from build123d import *

# Parameters (mm, degrees)
SKETCH1_R           = 150.5
BOSS_EXTRUDE1_DEPTH = 6.35
SKETCH3_R           = 2.6
CUT_EXTRUDE2_DEPTH  = 10
CUT_EXTRUDE3_DEPTH  = 10


with BuildPart() as part:
    # Sketch1 → Boss-Extrude1 (new body)
    # profile 1 of 2: a face of its own
    with BuildSketch(Plane(origin=(-388.281715987, 0, -288.185661777), x_dir=(1, 0, 0), z_dir=(0, 1, 0))):
        Polygon((1927.853460271, -13527.084883536), (1965.381699324, -13462.084066777), (1747.570833697, -13084.824581071), (1672.514355591, -13084.824581071), (1454.703489965, -13462.084066777), (1492.231729019, -13527.084883536), align=None)
        with Locations((1710.042594644, -13357.997843795)):
            Circle(SKETCH1_R, mode=Mode.SUBTRACT)
        with BuildLine():
            ThreePointArc((1909.99400131, -13496.418380494), (1909.919076, -13496.98749472), (1910.268520339, -13497.442899434))
            Line((1910.268520339, -13497.442899434), (1927.415821483, -13507.342898365))
            ThreePointArc((1927.415821483, -13507.342898365), (1927.984935702, -13507.417823673), (1928.440340423, -13507.068379346))
            Line((1928.440340423, -13507.068379346), (1948.340338275, -13472.600571997))
            ThreePointArc((1948.340338275, -13472.600571997), (1948.415263583, -13472.031457775), (1948.065819252, -13471.576053055))
            Line((1948.065819252, -13471.576053055), (1930.918518105, -13461.676054122))
            ThreePointArc((1930.918518105, -13461.676054122), (1930.349403886, -13461.601128813), (1929.893999164, -13461.95057314))
            Line((1929.893999164, -13461.95057314), (1909.99400131, -13496.418380494))
        make_face(mode=Mode.SUBTRACT)
        with BuildLine():
            ThreePointArc((1472.019370034, -13471.57605305), (1471.669925699, -13472.031457773), (1471.744851013, -13472.600571998))
            Line((1471.744851013, -13472.600571998), (1491.644848864, -13507.068379347))
            ThreePointArc((1491.644848864, -13507.068379347), (1492.100253585, -13507.41782368), (1492.669367808, -13507.342898369))
            Line((1492.669367808, -13507.342898369), (1509.816668952, -13497.442899438))
            ThreePointArc((1509.816668952, -13497.442899438), (1510.166113284, -13496.987494718), (1510.091187977, -13496.418380495))
            Line((1510.091187977, -13496.418380495), (1490.191190123, -13461.950573141))
            ThreePointArc((1490.191190123, -13461.950573141), (1489.735785404, -13461.60112881), (1489.166671181, -13461.676054117))
            Line((1489.166671181, -13461.676054117), (1472.019370034, -13471.57605305))
        make_face(mode=Mode.SUBTRACT)
        with BuildLine():
            ThreePointArc((1689.392596873, -13114.874577827), (1689.612266763, -13115.404907856), (1690.142596792, -13115.62457775))
            Line((1690.142596792, -13115.62457775), (1729.942592497, -13115.62457775))
            ThreePointArc((1729.942592497, -13115.62457775), (1730.472922528, -13115.404907859), (1730.692592416, -13114.874577827))
            Line((1730.692592416, -13114.874577827), (1730.692592416, -13095.074579966))
            ThreePointArc((1730.692592416, -13095.074579966), (1730.472922526, -13094.544249938), (1729.942592497, -13094.324580043))
            Line((1729.942592497, -13094.324580043), (1690.142596792, -13094.324580043))
            ThreePointArc((1690.142596792, -13094.324580043), (1689.612266761, -13094.544249935), (1689.392596873, -13095.074579966))
            Line((1689.392596873, -13095.074579966), (1689.392596873, -13114.874577827))
        make_face(mode=Mode.SUBTRACT)
    # profile 2 of 2: a face of its own
    with BuildSketch(Plane(origin=(-388.281715987, 0, -288.185661777), x_dir=(1, 0, 0), z_dir=(0, 1, 0))):
        with Locations((1710.042594644, -13357.997843795)):
            Circle(SKETCH1_R)
    extrude(amount=BOSS_EXTRUDE1_DEPTH)

    # Sketch3 → Cut-Extrude2 (cut)
    with BuildSketch(Plane(origin=(0, 6.35, 0), x_dir=(1, 0, 0), z_dir=(0, 1, 0))):
        with Locations(Location((1183.987460829, -12990.268662147, 0), (0, 0, 270))):
            Circle(SKETCH3_R)
        with Locations(Location((1146.487460829, -13055.220567431, 0), (0, 0, 270))):
            Circle(SKETCH3_R)
        with Locations(Location((1108.987460829, -13120.172472715, 0), (0, 0, 270))):
            Circle(SKETCH3_R)
        with Locations(Location((1221.487460829, -12925.316756863, 0), (0, 0, 270))):
            Circle(SKETCH3_R)
        with Locations(Location((1258.987460829, -12860.364851579, 0), (0, 0, 270))):
            Circle(SKETCH3_R)
        with Locations(Location((1459.534296487, -12990.268662148, 0), (0, 0, 270))):
            Circle(SKETCH3_R)
        with Locations(Location((1497.034296487, -13055.220567432, 0), (0, 0, 270))):
            Circle(SKETCH3_R)
        with Locations(Location((1534.534296487, -13120.172472716, 0), (0, 0, 270))):
            Circle(SKETCH3_R)
        with Locations(Location((1422.034296487, -12925.316756864, 0), (0, 0, 270))):
            Circle(SKETCH3_R)
        with Locations(Location((1384.534296487, -12860.364851581, 0), (0, 0, 270))):
            Circle(SKETCH3_R)
        with Locations(Location((1321.760878657, -13228.899221759, 0), (0, 0, 270))):
            Circle(SKETCH3_R)
        with Locations(Location((1246.760878657, -13228.899221759, 0), (0, 0, 270))):
            Circle(SKETCH3_R)
        with Locations(Location((1171.760878657, -13228.899221759, 0), (0, 0, 270))):
            Circle(SKETCH3_R)
        with Locations(Location((1396.760878657, -13228.899221759, 0), (0, 0, 270))):
            Circle(SKETCH3_R)
        with Locations(Location((1471.760878657, -13228.899221759, 0), (0, 0, 270))):
            Circle(SKETCH3_R)
    extrude(amount=-CUT_EXTRUDE2_DEPTH, mode=Mode.SUBTRACT)

    # Sketch4 → Cut-Extrude3 (cut)
    with BuildSketch(Plane(origin=(0, 6.35, 0), x_dir=(1, 0, 0), z_dir=(0, 1, 0))):
        with BuildLine():
            Line((1118.560623635, -13175.005548302), (1129.060623635, -13193.192081781))
            ThreePointArc((1129.060623635, -13193.192081781), (1130.275036352, -13194.123933434), (1131.792674443, -13193.924132589))
            Line((1131.792674443, -13193.924132589), (1139.327095456, -13189.574132589))
            ThreePointArc((1139.327095456, -13189.574132589), (1140.258947108, -13188.359719871), (1140.059146263, -13186.842081781))
            Line((1140.059146263, -13186.842081781), (1129.559146263, -13168.655548302))
            ThreePointArc((1129.559146263, -13168.655548302), (1128.344733546, -13167.723696649), (1126.827095456, -13167.923497494))
            Line((1126.827095456, -13167.923497494), (1119.292674443, -13172.273497494))
            ThreePointArc((1119.292674443, -13172.273497494), (1118.36082279, -13173.487910212), (1118.560623635, -13175.005548302))
        make_face()
        with BuildLine():
            Line((1332.260878658, -12841.23891597), (1311.260878658, -12841.23891597))
            ThreePointArc((1311.260878658, -12841.23891597), (1309.846665095, -12841.824702408), (1309.260878658, -12843.23891597))
            Line((1309.260878658, -12843.23891597), (1309.260878658, -12851.93891597))
            ThreePointArc((1309.260878658, -12851.93891597), (1309.846665095, -12853.353129533), (1311.260878658, -12853.93891597))
            Line((1311.260878658, -12853.93891597), (1332.260878658, -12853.93891597))
            ThreePointArc((1332.260878658, -12853.93891597), (1333.67509222, -12853.353129533), (1334.260878658, -12851.93891597))
            Line((1334.260878658, -12851.93891597), (1334.260878658, -12843.23891597))
            ThreePointArc((1334.260878658, -12843.23891597), (1333.67509222, -12841.824702408), (1332.260878658, -12841.23891597))
        make_face()
        with BuildLine():
            Line((1514.461133681, -13193.192081781), (1524.961133681, -13175.005548301))
            ThreePointArc((1524.961133681, -13175.005548301), (1525.160934526, -13173.487910211), (1524.229082873, -13172.273497494))
            Line((1524.229082873, -13172.273497494), (1516.69466186, -13167.923497494))
            ThreePointArc((1516.69466186, -13167.923497494), (1515.17702377, -13167.723696649), (1513.962611053, -13168.655548301))
            Line((1513.962611053, -13168.655548301), (1503.462611053, -13186.842081781))
            ThreePointArc((1503.462611053, -13186.842081781), (1503.262810208, -13188.359719871), (1504.19466186, -13189.574132588))
            Line((1504.19466186, -13189.574132588), (1511.729082873, -13193.924132588))
            ThreePointArc((1511.729082873, -13193.924132588), (1513.246720964, -13194.123933434), (1514.461133681, -13193.192081781))
        make_face()
    extrude(amount=-CUT_EXTRUDE3_DEPTH, mode=Mode.SUBTRACT)


solid = part.part
For this review, take the finished solid that the model builds, in its own axes (mm). A direction names the side the tool comes from. Round coordinates to 2 decimals unless told otherwise and drop trailing zeros. Write each loop counter-clockwise with the first axis right and the second up, starting at its lowest first coordinate (ties: lowest second). Pieces come first, ordered by that corner, then holes. Notation, with made-up numbers: M 27.25,83.25 L 63.25,83.25 A11 ccw 63.25,98.25 Z; hole C 76,52.5 d1. An arc over 180 degrees is marked long. Write item = value, one per line. Start each with the question number.
(1) We need section A-A (y = 3.25). Give the number of separate pieces and of enclosed holes in the cut face, then the cut area to 3 significant figures.
(2) We need section C-C (x = 1371). Give the boundary of the cut face in (y, z), then the cut area to 3 significant figures.
(3) Clearance check with flat-ended pins moving along their axes: pin 1 Ø3 at (y, z) = (3.5, 12848.5) entering from +X; pin 2 Ø3 at (x, z) = (1384.53, 12860.36) entering from +Y; pin 3 Ø1.5 at (x, y) = (1166, 2) entering from -Z. State where each tip first meets the part, or that it passes through.
(4) For line 1 along X through (y, z) = (2.75, 12923); line 2 along X through (y, z) = (3.5, 13179.5); line 3 along X through (y, z) = (3, 13216), list the stretches that pass through material, from the lowest coordinate up.
(5) We need section B-B (z = 12964). Give the boundary of the cut face in (x, y), then the cut area to 3 significant figures.
(6) The part is to be moulded in two halves that separate along Z. For faces 1 (the face through (1469.72, 3.13, 12987.91)), 2 (the face through (1531.8, 3.13, 13190.76)), 3 (the face through (1318, 0, 13064)), say which applies: +Z half, -Z half, draft (parallel to the pull), parting line (faces both ways), or undercut.
(7) For faces 4 (the face through (1519.638, 3.219, 13184.226)), 5 (the face through (1176.85, 3.13, 12982.63)), list the 3-axis set-ups (+Z, -Z, +X, -X, +Y, -Y) from which the entire face can be reached by the end or side of a thin tool; tool diameter is ignored.
Results found:
q1.separate_pieces = 1
q1.enclosed_holes = 21
q1.area = 137,000 mm²
q2.outline = M 0,12816.92 L 6.35,12816.92 L 6.35,13238.9 L 0,13238.9 Z
q2.area = 2,680 mm²
q3.pin_1 = 1390.1
q3.pin_2 = through
q3.pin_3 = 13000.12
q4.line_1 = 1211.28 to 1220.31, 1222.67 to 1420.85, 1423.21 to 1432.24
q4.line_2 = 1069.66 to 1090.48, 1105.22 to 1121.16, 1135.82 to 1507.7, 1522.37 to 1538.3, 1553.05 to 1573.87
q4.line_3 = 1090.73 to 1101.7, 1109.86 to 1533.67, 1541.82 to 1552.79
q5.outline = M 1187.61,0 L 1455.92,0 L 1455.92,6.35 L 1187.61,6.35 Z
q5.area = 1,700 mm²
q6.face_1 = -Z half
q6.face_2 = undercut
q6.face_3 = draft
q7.face_4 = +Y, -Y
q7.face_5 = -Z, -X, +Y, -Y
